from build123d import *

# Parameters (mm, degrees)
SKETCH1_W                  = 500
SKETCH1_H                  = 411.98
BOSS_EXTRUDE1_DEPTH        = 12
SKETCH2_W                  = 83.333333333
SKETCH2_H                  = 12
SKETCH2_W_2                = 12
SKETCH2_H_2                = 137.326666666
CUT_EXTRUDE1_DEPTH         = 12
SKETCH4_W                  = 12
SKETCH4_H                  = 24
SKETCH4_H_2                = 22
CUT_EXTRUDE2_DEPTH         = 12
SCALE1_SCALE               = 0.5
M2_5_START                 = 3
M2_5_CLEARANCE_SLOT1_DEPTH = 6
M3_CLEARANCE_SLOT1_D       = 3.4
M3_CLEARANCE_SLOT2_D       = 3.4


# Read off the part's stored shape, not the designer's step: M2.5 Clearance Slot1
with BuildPart() as part:
    # Sketch1 → Boss-Extrude1 (new body)
    with BuildSketch(Plane(origin=(0, 0, 0), x_dir=(1, 0, 0), z_dir=(0, 1, 0))):
        with Locations((250, 205.99)):
            Rectangle(SKETCH1_W, SKETCH1_H)
    extrude(amount=BOSS_EXTRUDE1_DEPTH)

    # Sketch2 → Cut-Extrude1 (cut)
    with BuildSketch(Plane(origin=(0, 12, 0), x_dir=(1, 0, 0), z_dir=(0, 1, 0))):
        with Locations((41.666666666, 6)):
            Rectangle(SKETCH2_W, SKETCH2_H)
        with Locations((458.333333334, 6)):
            Rectangle(SKETCH2_W, SKETCH2_H)
        with Locations((6, 205.99)):
            Rectangle(SKETCH2_W_2, SKETCH2_H_2)
        with Locations((494, 205.99)):
            Rectangle(SKETCH2_W_2, SKETCH2_H_2)
    extrude(amount=-CUT_EXTRUDE1_DEPTH, mode=Mode.SUBTRACT)

    # Sketch4 → Cut-Extrude2 (cut)
    with BuildSketch(Plane(origin=(0, 12, 0), x_dir=(1, 0, 0), z_dir=(0, 1, 0))):
        with Locations((6, 399.98)):
            Rectangle(SKETCH4_W, SKETCH4_H)
        with Locations((494, 399.98)):
            Rectangle(SKETCH4_W, SKETCH4_H)
        with Locations((494, 23)):
            Rectangle(SKETCH4_W, SKETCH4_H_2)
        with Locations((6, 24)):
            Rectangle(SKETCH4_W, SKETCH4_H)
    extrude(amount=-CUT_EXTRUDE2_DEPTH, mode=Mode.SUBTRACT)


with BuildPart() as part_1:
    # Scale1: scaled about (250.029343652, 6, -207.939049077)
    add(part.part.scale(SCALE1_SCALE).moved(Location((125.014671826, 3, -103.969524538))))

    # M2.5 Clearance Slot1 outline → M2.5 Clearance Slot1 (cut)
    with BuildSketch(Plane(origin=(0, 0, 0), x_dir=(1, 0, 0), z_dir=(0, 1, 0)).offset(M2_5_START)):
        with BuildLine():
            Line((138.354717143, 294.959902024), (138.454714786, 294.959215412))
            ThreePointArc((138.454714786, 294.959215412), (139.914636468, 296.399225372), (138.474626509, 297.859147054))
            Line((138.474626509, 297.859147054), (138.374628867, 297.859833665))
            ThreePointArc((138.374628867, 297.859833665), (136.914707184, 296.419823707), (138.354717143, 294.959902024))
        make_face()
        with BuildLine():
            Line((186.854717143, 293.859902024), (186.954714786, 293.859215412))
            ThreePointArc((186.954714786, 293.859215412), (188.414636468, 295.299225372), (186.974626509, 296.759147054))
            Line((186.974626509, 296.759147054), (186.874628867, 296.759833665))
            ThreePointArc((186.874628867, 296.759833665), (185.414707184, 295.319823707), (186.854717143, 293.859902024))
        make_face()
        with BuildLine():
            Line((168.754717143, 242.559902024), (168.854714786, 242.559215412))
            ThreePointArc((168.854714786, 242.559215412), (170.314636468, 243.999225372), (168.874626509, 245.459147054))
            Line((168.874626509, 245.459147054), (168.774628867, 245.459833665))
            ThreePointArc((168.774628867, 245.459833665), (167.314707184, 244.019823707), (168.754717143, 242.559902024))
        make_face()
        with BuildLine():
            Line((142.954717143, 242.559902024), (143.054714786, 242.559215412))
            ThreePointArc((143.054714786, 242.559215412), (144.514636468, 243.999225372), (143.074626509, 245.459147054))
            Line((143.074626509, 245.459147054), (142.974628867, 245.459833665))
            ThreePointArc((142.974628867, 245.459833665), (141.514707184, 244.019823707), (142.954717143, 242.559902024))
        make_face()
    extrude(amount=M2_5_CLEARANCE_SLOT1_DEPTH, mode=Mode.SUBTRACT)

    # M3 Clearance Slot1 (through all)
    with Locations(Plane(origin=(0, 9, 0), x_dir=(1, 0, 0), z_dir=(0, 1, 0))):
        with Locations((200.214671826, 226.059524539), (200.214671826, 284.659524539), (249.814671826, 284.659524539), (249.814671826, 226.059524539), (235.514671826, 116.964788111), (288.014671826, 185.464788111), (330.514671826, 116.964788111), (290.914671826, 205.488524539), (291.144671826, 291.089524539), (351.524671826, 281.939524539), (350.704671826, 204.749524539), (302.114671826, 304.959524539), (347.014671826, 304.959524539)):
            Hole(M3_CLEARANCE_SLOT1_D / 2)

    # M3 Clearance Slot2 (through all)
    with Locations(Plane(origin=(0, 3, 0), x_dir=(-1, 0, 0), z_dir=(0, -1, 0))):
        with Locations((-372.014671826, 137.856191205), (-372.014671826, 155.746191205), (-372.014671826, 260.182857872), (-372.014671826, 279.072857872), (-128.014671826, 138.856191205), (-128.014671826, 155.746191205), (-128.014671826, 260.182857872), (-128.014671826, 279.072857872)):
            Hole(M3_CLEARANCE_SLOT2_D / 2)


solid = part_1.part
CAD build for the part. Positions are in the model's coordinates, mm. A direction names the side the tool comes from. Give positions to 0.01 mm unless a question says otherwise; leave off trailing zeros. Write each loop counter-clockwise with the first axis right and the second up, starting at its lowest first coordinate (ties: lowest second). Pieces come first, ordered by that corner, then holes. Notation, with made-up numbers: (2.5, 68.5) -> (28.5, 68.5) arc R16 cw to (28.5, 83.5) -> close; hole circle Ø11 at (25.25, 42.5). An arc over 180 degrees is marked (long way). Return JSON: item names as keys, results as strings.
Item 1: Band-saw the part on A-A (z = -214). List the corners of the cut face in (x, y).
Answer below:
{"outline": "(131.01, 3) -> (369.01, 3) -> (369.01, 9) -> (131.01, 9) -> close"}
Item 2: Drop flat-ended pins along their axis: pin 1 (1.8 mm diameter, centred on x = 128.5, y = 6.5, fed in from -Z); pin 2 (3 mm diameter, centred on y = 7, z = -216.5, fed in from -X); pin 3 (2 mm diameter, centred on x = 350.7, z = -204.75, fed in from -Y); pin 4 (3 mm diameter, centred on x = 346, y = 4.5, fed in from +Z). Give the stop position or say it passes through.
Answer below:
{"pin 1": "stops at z = -297.96", "pin 2": "stops at x = 131.01", "pin 3": "passes through", "pin 4": "stops at z = -109.97"}
Item 3: Drill centre lines: probe 1 along X at (y, z) = (5.5, -284.5); probe 2 along Z at (x, y) = (358, 6.9); probe 3 along Z at (x, y) = (331, 7.25). Where is each one in solid material? Low to high.
Answer below:
{"probe 1": "x = 125.01 to 198.52, 201.91 to 248.12, 251.51 to 375.01", "probe 2": "z = -309.96 to -109.97", "probe 3": "z = -309.96 to -118.59, -115.34 to -103.97"}
Item 4: Band-saw the part on B-B (y = 6.95). Give the number of separate pieces and of enclosed holes in the cut face, then the cut area to 3 significant figures.
Answer below:
{"separate pieces": "1", "enclosed holes": "25", "area": "49,700 mm2"}
Item 5: Two-plate mould, pull along Z, no slides. Class faces 5 (the flat face through (372, 6, -172.633)), 6 (the flat face through (131.015, 6, -304)), 7 (the flat face through (249, 6, -103.97)): +Z half, -Z half, draft (parallel to the pull), parting line (faces both ways), or undercut.
Answer below:
{"face 5": "undercut", "face 6": "draft", "face 7": "+Z half"}
Item 6: Tool access for faces 1 (the flat face through (351, 6, -109.97)), 2 (the flat face through (128, 6, -121.97)), 3 (the flat face through (372, 6, -241.296)), 4 (the flat face through (128, 6, -297.96)): list every direction of +Z, -Z, +X, -X, +Y, -Y with a clear straight run to the whole face (end or side of a thin tool).
Answer below:
{"face 1": "+Z, +X, +Y, -Y", "face 2": "+Z, -X, +Y, -Y", "face 3": "+X, +Y, -Y", "face 4": "-Z, -X, +Y, -Y"}
